Autodesk Inventor part; units mm, degrees
ref_plane "YZ Plane" through (0, 0, 0) normal (1, 0, 0) x (0, 1, 0)
ref_plane "XZ Plane" through (0, 0, 0) normal (0, 1, 0) x (-1, 0, 0)
ref_plane "XY Plane" through (0, 0, 0) normal (0, 0, 1) x (1, 0, 0)
ref_plane "Work Plane1" through (0, 0, 0) normal (0, 0, 1) x (1, 0, 0)
sketch "Sketch1" plane through (0, 0, 0) normal (0, 0, 1) x (1, 0, 0)
  line L0 (88.9, -98.425) -> (-88.9, -98.425)
  line L1 (-88.9, -98.425) -> (-88.9, -28.575)
  line L2 (-88.9, -28.575) -> (-88.9, 28.575)
  line L3 (-88.9, 28.575) -> (-85.09, 28.575)
  line L4 (88.9, 28.575) -> (88.9, -28.575)
  line L5 (85.09, 28.575) -> (88.9, 28.575)
  line L6 (88.9, -28.575) -> (88.9, -98.425)
  line L7 (-88.9, 28.575) -> (88.9, 28.575)
  line L8 (88.9, 28.575) -> (88.9, -98.425)
  line L9 (88.9, -98.425) -> (-88.9, -98.425)
  line L10 (-88.9, -98.425) -> (-88.9, 28.575)
  point P0 (0, 0)
extrude "Extrusion1" add sketch "Sketch1" along normal blind 6.35
sketch "Sketch2" plane through (0, 0, 6.35) normal (0, 0, 1) x (1, 0, 0)
  line L0 (-88.9, -98.425) -> (88.9, -98.425)
  line L1 (-88.9, -98.425) -> (-88.9, -28.575)
  line L2 (-88.9, 28.575) -> (-88.9, -98.425)
  line L3 (88.9, -98.425) -> (88.9, 28.575)
  circle A0 centre (-44.45, -80.9625) radius 3.937
  line L4 (-88.9, 28.575) -> (88.9, 28.575)
  line L5 (88.9, 28.575) -> (88.9, -28.575)
  line L6 (88.9, -28.575) -> (-88.9, -28.575)
  line L7 (-88.9, -28.575) -> (-88.9, 28.575)
  line L8 (88.9, 28.575) -> (-88.9, 28.575)
  line L9 (0, 28.575) -> (0, -28.575)
  line L10 (-66.675, -80.9625) -> (-44.45, -80.9625)
  line L11 (-55.5874, 4.1336) -> (-33.3126, 4.1336)
  line L12 (-33.3126, 4.1336) -> (-33.3126, -4.1336)
  line L13 (-33.3126, -4.1336) -> (-55.5874, -4.1336)
  line L14 (-55.5874, -4.1336) -> (-55.5874, 4.1336)
  line L15 (-55.5874, 4.1336) -> (-33.3126, -4.1336) construction
  line L16 (-33.3126, 4.1336) -> (-55.5874, -4.1336) construction
  line L17 (34.2724, -7.1205) -> (54.0224, -7.1205)
  line L18 (54.0224, -7.1205) -> (54.0224, -24.7205)
  line L19 (54.0224, -24.7205) -> (34.2724, -24.7205)
  line L20 (34.2724, -24.7205) -> (34.2724, -7.1205)
  line L21 (34.2724, -7.1205) -> (54.0224, -24.7205) construction
  line L22 (54.0224, -7.1205) -> (34.2724, -24.7205) construction
  line L23 (39.3724, 16.9458) -> (54.0224, 16.9458)
  line L24 (54.0224, 16.9458) -> (54.0224, 0.4458)
  line L25 (54.0224, 0.4458) -> (39.3724, 0.4458)
  line L26 (39.3724, 0.4458) -> (39.3724, 16.9458)
  line L27 (39.3724, 16.9458) -> (54.0224, 0.4458) construction
  line L28 (54.0224, 16.9458) -> (39.3724, 0.4458) construction
  point P0 (0, 0)
  point P1 (44.1474, -15.9205)
  point P2 (46.6974, 8.6958)
  dimension "d2" = 69.85
  dimension "d5" = 7.874
  dimension "d8" = 22.2748
  dimension "d9" = 8.2672
  dimension "d10" = 16.5
  dimension "d11" = 14.65
  dimension "d12" = 19.75
  dimension "d13" = 17.6
extrude "Extrusion2" cut sketch "Sketch2" against normal through all contours A0 | L11 L12 L13 L14 | L17 L18 L19 L20 | L23 L24 L25 L26
sketch "Sketch3" plane through (0, 0, 6.35) normal (0, 0, 1) x (1, 0, 0)
  line L0 (88.9, 28.575) -> (-88.9, 28.575)
  line L1 (-88.9, -98.425) -> (88.9, -98.425)
  line L2 (-88.9, -98.425) -> (88.9, -98.425)
  line L3 (0, 25.29) -> (30.48, 25.29) construction
  line L4 (0, 25.29) -> (-2.1566, 0.6394)
  line L5 (0, 25.29) -> (24.7447, 25.29) construction
  line L6 (-2.1566, 0.6394) -> (0, -24.0111)
  line L7 (0, -24.0111) -> (2.1566, -48.6616)
  line L8 (2.1566, -48.6616) -> (0, -73.3121)
  line L9 (0, -73.3121) -> (-2.1566, -97.9626)
  line L10 (0, 25.29) -> (0, 28.575)
  line L11 (-2.1566, -97.9626) -> (-2.1566, -98.425)
  line L12 (-88.9, 28.575) -> (-88.9, -98.425)
  line L13 (-33.3126, -4.1336) -> (-55.5874, -4.1336)
  line L14 (-55.5874, -4.1336) -> (-55.5874, 4.1336)
  line L15 (-55.5874, 4.1336) -> (-33.3126, 4.1336)
  line L16 (-33.3126, 4.1336) -> (-33.3126, -4.1336)
  line L17 (54.0224, -7.1205) -> (54.0224, -24.7205)
  line L18 (54.0224, -24.7205) -> (34.2724, -24.7205)
  line L19 (34.2724, -24.7205) -> (34.2724, -7.1205)
  line L20 (34.2724, -7.1205) -> (54.0224, -7.1205)
  circle A0 centre (-44.45, -80.9625) radius 3.937
  line L21 (39.3724, 0.4458) -> (39.3724, 16.9458)
  line L22 (39.3724, 16.9458) -> (54.0224, 16.9458)
  line L23 (54.0224, 16.9458) -> (54.0224, 0.4458)
  line L24 (54.0224, 0.4458) -> (39.3724, 0.4458)
  line L25 (88.9, 28.575) -> (-88.9, 28.575)
  line L26 (-88.9, 28.575) -> (-88.9, -98.425)
  line L27 (-88.9, -98.425) -> (88.9, -98.425)
  line L28 (88.9, -98.425) -> (88.9, 28.575)
  point P0 (0, 0)
  dimension "d21" = 24.7447
  dimension "d22" = 95
  dimension "d23" = 24.7447
  dimension "d24" = 24.7447
  dimension "d25" = 180
  dimension "d26" = 24.7447
  dimension "d27" = 24.7447
extrude "Extrusion5" cut sketch "Sketch3" against normal blind 25.4 contours L28 L1 L11 L9 L8 L7 L6 L4 L10 L0
properties part number "compnent box front L"
Geometry: final body of the model. Coordinates: model frame, mm. A direction names the side the tool comes from. Coordinates: 2 decimals unless noted, no trailing zeros. Order: outer loops, then holes, each group sorted by start corner. A loop starts at its lowest first (then second) coordinate and runs counter-clockwise, first axis right, second up. Notation, with made-up numbers: (19, -27) - (27, -27) arc R7 ccw to (27, -22) - close; hole circle Ø8 at (72, -34.5). An arc over 180 degrees is marked (long way). Return JSON: item names as keys, results as strings. Group by question number.
1. Pin query (flat end, axial travel): pin 1 (2.5 mm diameter, centred on y = 26.5, z = 3.5, fed in from +X). Return the tip coordinate at first contact, or that it passes through.
2. Material intervals for line 1 along Y through (x, z) = (-44.45, 2.75) (1 decimal); line 2 along Y through (x, z) = (-35, 5) (3 decimals); line 3 along Y through (x, z) = (-46, 5.5) (3 decimals), sorted ascending. Write a range as [from, to].
3. Cut plane D-D (y = 20). Output: boundary loops of the cut face in (x, z), plus the area to 3 significant figures.
4. Cut plane A-A (x = -44.45). Count the separate pieces of the cut face and the enclosed holes in it, plus the area to 3 significant figures.
5. Pull-direction query (Y, two-part tool) for faces 1 (the face through (-44, -34, 0)), 2 (the face through (0.03, -72.97, 3.22)), 3 (the face through (0, -24, 3)); classes: pulls with the +Y half, pulls with the -Y half, needs draft (parallel to the pull), parting line crosses it, or undercut.
6. Set-up query: faces 4 (the face through (0, 27, 3)), 5 (the face through (-45, -98.425, 3)), 6 (the face through (-1.063, 13.137, 3.219)), 7 (the face through (-44, -34, 6.35)), 8 (the face through (-55.587, 0, 3)). Return all of +Z, -Z, +X, -X, +Y, -Y with unobstructed straight access to the full face (end or side cutting, diameter ignored); none if empty.
7. Cut plane C-C (y = -32.5). Output: boundary loops of the cut face in (x, z), plus the area to 3 significant figures.
Resolved:
{
 "1": {"pin 1": "stops at x = 0"},
 "2": {"line 1": "y = [-98.4, -84.9], [-77, -4.1], [4.1, 28.6]", "line 2": "y = [-98.425, -4.134], [4.134, 28.575]", "line 3": "y = [-98.425, -84.582], [-77.343, -4.134], [4.134, 28.575]"},
 "3": {"outline": "(-88.9, 0) - (-0.46, 0) - (-0.46, 6.35) - (-88.9, 6.35) - close", "area": "562 mm²"},
 "4": {"separate pieces": "3", "enclosed holes": "0", "area": "704 mm²"},
 "5": {"face 1": "needs draft", "face 2": "pulls with the -Y half", "face 3": "undercut"},
 "6": {"face 4": "+Z, -Z, +X, +Y", "face 5": "+Z, -Z, +X, -X, -Y", "face 6": "+Z, -Z, +X", "face 7": "+Z, +X, -X, +Y, -Y", "face 8": "+Z, -Z"},
 "7": {"outline": "(-88.9, 0) - (0.74, 0) - (0.74, 6.35) - (-88.9, 6.35) - close", "area": "569 mm²"}
}
